For this review, take the finished solid that the model builds, in its own axes (mm). Face numbers are marked on the shaded views. A direction names the side the tool comes from. Coordinates: 2 decimals unless noted, no trailing zeros. Order: outer loops, then holes, each group sorted by start corner. A loop starts at its lowest first (then second) coordinate and runs counter-clockwise, first axis right, second up. Notation, with made-up numbers: (-10, 37.5) -> (37, 37.5) arc R21 ccw to (37, 41.5) -> close; hole circle Ø4 at (-37.5, -13.5). An arc over 180 degrees is marked (long way). Answer as a JSON object with one key per item and string values. Group by question number.
1) Add section D-D, the plane z = -6.5. Write out the cut boundary in (x, y), then the cut area to 3 significant figures.
2) Add section C-C, the plane y = -6. Write out the cut boundary in (x, z).
3) Wall thickness on L1, parallel to X at y = 4, z = -8; L2, parallel to Y at x = -21.5, z = -2.5; L3, parallel to Y at x = 33.5, z = 1: over which ranges is each line inside the solid? List them lowest first.
4) Machinability: for the marked faces 1 and 2, which of the approach directions +Z, -Z, +X, -X, +Y, -Y give a long, thin tool a straight path to every point of the face, cutting with its end or side? Answer none if there is none.
5) Add section A-A, the plane z = 0. Write out the cut boundary in (x, y).
6) Add section B-B, the plane x = -20. Write out the cut boundary in (y, z).
7) For pin 1 (4 mm diameter, centred on x = -12, y = 18.5, fed in from +Z); pin 2 (10 mm diameter, centred on y = 13, z = -4, fed in from +X); pin 3 (4 mm diameter, centred on x = -17, y = 18, fed in from -Z), all flat-tipped, find the tip position at first contact; note any pin that passes through.
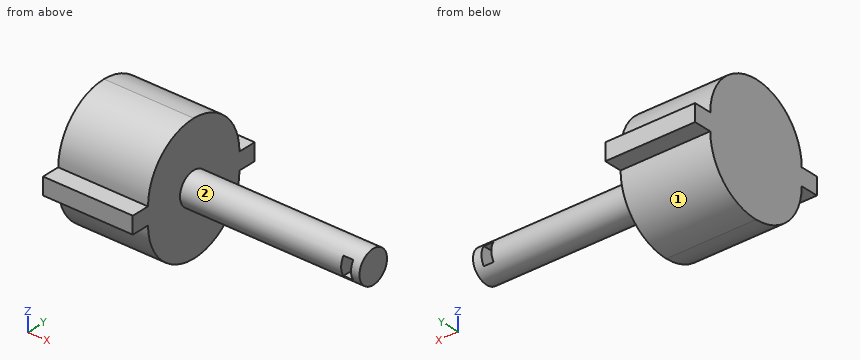
from build123d import *

# Parameters (mm, degrees)
F0_W        = 29.9085080624
F0_H        = 34.6928238869
F1_DEPTH    = 25
F2_R        = 4.5021693383
F3_DEPTH    = 50
F4_T1_DEPTH = 100
F5_DEPTH    = 5
F6_DEPTH    = 5
F8_DEPTH    = 2.5


# Not quite as in the source:
# - a fillet or chamfer that OpenCascade refuses, or shapes differently, is made with other operations: its cross-section is extruded or revolved along the edge and cut away or added


with BuildPart() as f1:
    # F0 (on Right) → F1 (new body)
    with BuildSketch(Plane.YZ):
        Rectangle(F0_W, F0_H)
    extrude(amount=-F1_DEPTH)

    # F2 (on Right) → F3 (join)
    with BuildSketch(Plane.YZ):
        Circle(F2_R)
    extrude(amount=F3_DEPTH)

    # F4: fillet of radius 15 on 4 edges, made by hand

    # F4_s2 → F4_t1 (cut)
    with BuildSketch(Plane.YZ.offset(-62.5)):
        with BuildLine():
            ThreePointArc((0.0457459688, 17.3464119434), (-10.560855749, 12.9530136612), (-14.9542540312, 2.3464119434))
            Line((-14.9542540312, 2.3464119434), (-14.9542540312, 17.3464119434))
            Line((-14.9542540312, 17.3464119434), (0.0457459688, 17.3464119434))
        make_face()
        with BuildLine():
            ThreePointArc((14.9542540312, -2.3464119434), (10.560855749, -12.9530136612), (-0.0457459688, -17.3464119434))
            Line((-0.0457459688, -17.3464119434), (14.9542540312, -17.3464119434))
            Line((14.9542540312, -17.3464119434), (14.9542540312, -2.3464119434))
        make_face()
        with BuildLine():
            ThreePointArc((14.9542540312, 2.3464119434), (10.560855749, 12.9530136612), (-0.0457459688, 17.3464119434))
            Line((-0.0457459688, 17.3464119434), (14.9542540312, 17.3464119434))
            Line((14.9542540312, 17.3464119434), (14.9542540312, 2.3464119434))
        make_face()
        with BuildLine():
            ThreePointArc((0.0457459688, -17.3464119434), (-10.560855749, -12.9530136612), (-14.9542540312, -2.3464119434))
            Line((-14.9542540312, -2.3464119434), (-14.9542540312, -17.3464119434))
            Line((-14.9542540312, -17.3464119434), (0.0457459688, -17.3464119434))
        make_face()
    extrude(amount=F4_T1_DEPTH, mode=Mode.SUBTRACT)

    # F5 (add): a face of the model
    f5_faces = [f1.faces().sort_by_distance(p)[0] for p in [
        (-12.5, 14.9542540312, 0),
    ]]
    extrude(f5_faces, amount=F5_DEPTH)

    # F6 (add): a face of the model
    f6_faces = [f1.faces().sort_by_distance(p)[0] for p in [
        (-12.5, -14.9542540312, 0),
    ]]
    extrude(f6_faces, amount=F6_DEPTH)

    # F7 (on Top) → F8 (cut, symmetric)
    with BuildSketch(Plane.XY):
        Polygon((44.8985174298, 7.189091295), (44.8985174298, -8.9538004249), (47.6411059499, -8.9538004249), (47.6411059499, 6.886465475), align=None)
    extrude(amount=F8_DEPTH, both=True, mode=Mode.SUBTRACT)


solid = f1.part
Output values:
{
 "1": {"outline": "(-25, -14.37) -> (0, -14.37) -> (0, 14.37) -> (-25, 14.37) -> close", "area": "718 mm²"},
 "2": {"outline": "(-25, -16.07) -> (0, -16.07) -> (0, 16.07) -> (-25, 16.07) -> close"},
 "3": {"L1": "x = -25 to 0", "L2": "y = -14.95 to 14.95", "L3": "y = -4.39 to 4.39"},
 "4": {"face 1": "-Z, +X, -X, +Y", "face 2": "+X"},
 "5": {"outline": "(-25, -19.95) -> (0, -19.95) -> (0, -4.5) -> (44.9, -4.5) -> (44.9, 4.5) -> (0, 4.5) -> (0, 19.95) -> (-25, 19.95) -> close; (47.64, -4.5) -> (50, -4.5) -> (50, 4.5) -> (47.64, 4.5) -> close"},
 "6": {"outline": "(-19.95, -2.35) -> (-14.95, -2.35) arc R15 ccw to (0, -17.35) arc R15 ccw to (14.95, -2.35) -> (19.95, -2.35) -> (19.95, 2.35) -> (14.95, 2.35) arc R15 ccw to (0, 17.35) arc R15 ccw to (-14.95, 2.35) -> (-19.95, 2.35) -> close"},
 "7": {"pin 1": "stops at z = 2.35", "pin 2": "stops at x = 0", "pin 3": "stops at z = -2.35"}
}
